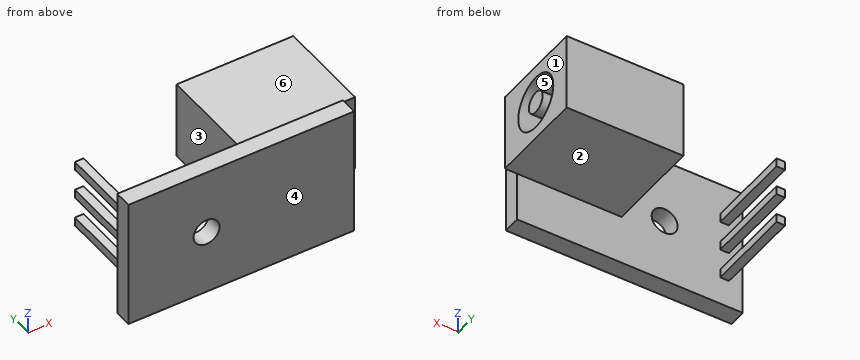
```python
from build123d import *

# Parameters (mm, degrees)
SKETCH1_W           = 26
SKETCH1_H           = 15
BOSS_EXTRUDE1_DEPTH = 2
SKETCH2_W           = 13.45020195
SKETCH2_H           = 9
BOSS_EXTRUDE2_DEPTH = 11
SKETCH3_R           = 1.5
CUT_EXTRUDE1_DEPTH  = 11
SKETCH4_W           = 1
SKETCH4_H           = 1
BOSS_EXTRUDE3_DEPTH = 10
SKETCH5_R           = 3.118355213
SKETCH5_R_2         = 1.2290481
CUT_EXTRUDE2_DEPTH  = 10


with BuildPart() as part:
    # Sketch1 → Boss-Extrude1 (new body)
    with BuildSketch(Plane(origin=(0, 0, 0), x_dir=(1, 0, 0), z_dir=(0, 1, 0))):
        Rectangle(SKETCH1_W, SKETCH1_H)
    extrude(amount=BOSS_EXTRUDE1_DEPTH)

    # Sketch2 → Boss-Extrude2 (add)
    with BuildSketch(Plane(origin=(0, 2, 0), x_dir=(1, 0, 0), z_dir=(0, 1, 0))):
        with Locations((7.687739683, -2.759900257)):
            Rectangle(SKETCH2_W, SKETCH2_H)
    extrude(amount=BOSS_EXTRUDE2_DEPTH)

    # Sketch3 → Cut-Extrude1 (cut)
    with BuildSketch(Plane(origin=(0, 2, 0), x_dir=(1, 0, 0), z_dir=(0, 1, 0))):
        with Locations(Location((-4, 0, 0), (0, 0, 270))):
            Circle(SKETCH3_R)
    extrude(amount=-CUT_EXTRUDE1_DEPTH, mode=Mode.SUBTRACT)

    # Sketch4 → Boss-Extrude3 (add)
    with BuildSketch(Plane(origin=(0, 2, 0), x_dir=(1, 0, 0), z_dir=(0, 1, 0))):
        with Locations((-10.910563353, -3.293392003)):
            Rectangle(SKETCH4_W, SKETCH4_H)
        with Locations((-10.910563353, 0.206607997)):
            Rectangle(SKETCH4_W, SKETCH4_H)
        with Locations((-10.910563353, 3.706607997)):
            Rectangle(SKETCH4_W, SKETCH4_H)
    extrude(amount=BOSS_EXTRUDE3_DEPTH)

    # Sketch5 → Cut-Extrude2 (cut)
    with BuildSketch(Plane(origin=(14.412840658, 0, 0), x_dir=(0, 0, -1), z_dir=(1, 0, 0))):
        with Locations((-2.759900257, 7.5)):
            Circle(SKETCH5_R)
        with Locations((-2.759900257, 7.5)):
            Circle(SKETCH5_R_2, mode=Mode.SUBTRACT)
    extrude(amount=-CUT_EXTRUDE2_DEPTH, mode=Mode.SUBTRACT)


solid = part.part
```
Verification items for the finished model (mm, model axes). Face numbers are marked on the shaded views. A direction names the side the tool comes from. Coordinates: 2 decimals unless noted, no trailing zeros. Write each loop counter-clockwise with the first axis right and the second up, starting at its lowest first coordinate (ties: lowest second). Pieces come first, ordered by that corner, then holes. Notation, with made-up numbers: M -26.5,22 L 6.5,22 A18 ccw 6.5,38 Z; hole C 60.5,40.5 d1. An arc over 180 degrees is marked long. Answer as a JSON object with one key per item and string values. Group by question number.
(1) Cross-section at C-C, the plane x = -4. Record the cut outline in (y, z).
(2) Cross-section at D-D, the plane z = 0. Record the cut outline in (x, y), and give its area (3 significant figures).
(3) Gauge pin test, flat ends, axial feed: pin 1 (4.5 mm diameter, centred on x = -1, z = -3, fed in from +Y); pin 2 (0.5 mm diameter, centred on x = -11, y = 7, fed in from +Z); pin 3 (5 mm diameter, centred on x = -0.5, y = 9.5, fed in from -Z); pin 4 (1.8 mm diameter, centred on x = -4, z = 0, fed in from +Y). Record the tip position at first contact, or that the pin passes through.
(4) Cross-section at A-A, the plane x = 12. Record the cut outline in (y, z), and give its area (3 significant figures).
(5) Cross-section at B-B, the plane y = 11. Record the cut outline in (x, z).
(6) Material ranges on line 1 (X direction, y = 1.5, z = 0); line 2 (X direction, y = 7, z = 3.5); line 3 (Y direction, x = -5.5, z = 6.5), recorded low to high.
(7) Release check for a two-part mould opening along X. For the marked faces 1, 2 and 3 record: +X half, -X half, draft (parallel to the pull), parting line (faces both ways), or undercut.
(8) Tool access check on the marked faces 4, 5 and 6. Record the directions out of +Z, -Z, +X, -X, +Y, -Y that give a thin tool (end or side, any length) a straight path to the whole face; none if there is none.
Reply:
{
 "1": {"outline": "M 0,-7.5 L 2,-7.5 L 2,-1.5 L 0,-1.5 Z; M 0,1.5 L 2,1.5 L 2,7.5 L 0,7.5 Z"},
 "2": {"outline": "M -13,0 L -5.5,0 L -5.5,2 L -10.41,2 L -10.41,12 L -11.41,12 L -11.41,2 L -13,2 Z; M -2.5,0 L 13,0 L 13,2 L 14.41,2 L 14.41,6.05 L 4.41,6.05 L 4.41,8.95 L 14.41,8.95 L 14.41,13 L 0.96,13 L 0.96,2 L -2.5,2 Z", "area": "175 mm²"},
 "3": {"pin 1": "y = 2", "pin 2": "z = 3.79", "pin 3": "z = -1.74", "pin 4": "through"},
 "4": {"outline": "M 0,-7.5 L 2,-7.5 L 2,-1.74 L 13,-1.74 L 13,7.26 L 2,7.26 L 2,7.5 L 0,7.5 Z; C 7.5,2.76 d2.46; hole C 7.5,2.76 d6.24", "area": "103 mm²"},
 "5": {"outline": "M -11.41,-4.21 L -10.41,-4.21 L -10.41,-3.21 L -11.41,-3.21 Z; M -11.41,-0.71 L -10.41,-0.71 L -10.41,0.29 L -11.41,0.29 Z; M -11.41,2.79 L -10.41,2.79 L -10.41,3.79 L -11.41,3.79 Z; M 0.96,-1.74 L 14.41,-1.74 L 14.41,7.26 L 0.96,7.26 Z"},
 "6": {"line 1": "-13 to -5.5, -2.5 to 13", "line 2": "-11.41 to -10.41, 0.96 to 14.41", "line 3": "0 to 2"},
 "7": {"face 1": "+X half", "face 2": "draft", "face 3": "undercut"},
 "8": {"face 4": "+Z, -Z, +X, -X, -Y", "face 5": "+X", "face 6": "+Z, +X, -X, +Y"}
}
